Autodesk Inventor part; units mm, degrees
ref_plane "YZ Plane" through (0, 0, 0) normal (1, 0, 0) x (0, 1, 0)
ref_plane "XZ Plane" through (0, 0, 0) normal (0, 1, 0) x (-1, 0, 0)
ref_plane "XY Plane" through (0, 0, 0) normal (0, 0, 1) x (1, 0, 0)
sketch "Szkic1" plane through (0, 0, 0) normal (0, 1, 0) x (-1, 0, 0)
  line L0 (0, 0) -> (0, -97)
  line L1 (0, -97) -> (70, -97)
  line L2 (70, -97) -> (70, 0)
  line L3 (70, 0) -> (0, 0)
  line L4 (70, 0) -> (85, 0)
  line L5 (85, 0) -> (85, -97)
  line L6 (85, -97) -> (70, -97)
  line L7 (0, -97) -> (-15, -97)
  line L8 (-15, -97) -> (-15, 0)
  line L9 (-15, 0) -> (0, 0)
  line L10 (70, 0) -> (70, -25)
  line L11 (70, -25) -> (0, -25)
  line L12 (70, -97) -> (70, -72)
  line L13 (70, -72) -> (0, -72)
  line L14 (70, -48.5) -> (70, -72.5)
  line L15 (70, -48.5) -> (70, -24.5)
  line L16 (0, -48.5) -> (0, -72.5)
  line L17 (0, -48.5) -> (0, -24.5)
  dimension "d0" = 97
  dimension "d1" = 70
  dimension "d2" = 15
  dimension "d3" = 15
  dimension "d4" = 25
  dimension "d5" = 25
  dimension "d6" = 24
  dimension "d7" = 24
  dimension "d8" = 24
  dimension "d9" = 24
extrude "Wyciągnięcie proste1" add sketch "Szkic1" along normal blind 40 contours L0 L7 L8 L9 | L4 L5 L6 L2
sketch "Szkic2" plane through (0, 40, 0) normal (0, 1, 0) x (1, 0, 0)
  point P0 (0, 0)
sketch "Szkic3" plane through (0, 0, 0) normal (0, -1, 0) x (1, 0, 0)
  line L0 (-70, 0) -> (-70, -97)
  line L1 (-70, 0) -> (-70, -22)
  line L2 (-70, -22) -> (0, -22)
  line L3 (0, -97) -> (0, 0)
  line L4 (0, -22) -> (0, 0)
  line L5 (0, 0) -> (-70, 0)
  line L6 (-70, -97) -> (-70, -75)
  line L7 (-70, -75) -> (0, -75)
  line L8 (0, -97) -> (-70, -97)
  dimension "d12" = 22
  dimension "d13" = 22
extrude "Wyciągnięcie proste2" add sketch "Szkic3" against normal blind 30 contours L5 L3 L2 L0 | L7 L3 L8 L0
sketch "Szkic4" plane through (-85, 0, -97) normal (-1, 0, 0) x (0, 0, 1)
  line L0 (0, 0) -> (97, 0)
  line L1 (0, 0) -> (48.5, 0)
  line L2 (48.5, 0) -> (72.5, 0)
  line L3 (75, 0) -> (22, 0)
  line L4 (48.5, 0) -> (24.5, 0)
  line L5 (0, 0) -> (0, 40)
  line L6 (24.5, 0) -> (0, 0)
  line L7 (24.5, 0) -> (24.5, 15.2326)
  line L8 (24.5, 0) -> (39.7326, 0) construction
  line L9 (24.5, 0) -> (24.5, 20)
  circle A0 centre (24.5, 20) radius 20
  line L10 (24.5, 20) -> (72.5, 20)
  circle A1 centre (72.5, 20) radius 20
  dimension "d16" = 48.5
  dimension "d17" = 24
  dimension "d18" = 24
  dimension "d19" = 90
  dimension "d20" = 20
  dimension "d21" = 48
properties part number "podwozie"
Design review of the part built by this model. Coordinates are the model's own, in mm. A direction names the side the tool comes from. Coordinates: 2 decimals unless noted, no trailing zeros. Loops run counter-clockwise (first coordinate to the right, second up) from the corner with the lowest first, then second, coordinate; pieces in that order, holes last. Notation, with made-up numbers: (15, 32) - (74, 32) arc R17 ccw to (74, 45) - close; hole circle Ø11 at (77, 24). An arc over 180 degrees is marked (long way). Use CSV: the item, a comma, the result in double quotes. Start each with the question number.
1. Add section D-D on z = -13. Give the boundary of the cut face in (x, y).
2. Add section B-B on z = -63. Give the boundary of the cut face in (x, y), plus the area to 3 significant figures.
3. For faces 1 (the flat face through (-35, 30, -11)), 2 (the flat face through (0, 24, -48)), 3 (the flat face through (-34, 15, 0)), 4 (the flat face through (-35, 15, -75)), list the 3-axis set-ups (+Z, -Z, +X, -X, +Y, -Y) from which the entire face can be reached by the end or side of a thin tool; tool diameter is ignored.
4. Add section A-A on x = -67.5. Give the boundary of the cut face in (y, z).
5. Mouldability with a two-part tool opening along Z and no side actions: class faces 5 (the flat face through (-35, 15, -22)), 6 (the flat face through (15, 20, -49)), 7 (the flat face through (-70, 24, -49)), 8 (the flat face through (-36, 15, -97)) as released by +Z, released by -Z, zero draft, split by the parting line, or undercut.
6. Clearance check with a flat-ended pin moving along its axis: pin 1 (2 mm diameter, centred on x = -48.5, z = -86.5, fed in from +Y). State where the tip first meets the part, or that it passes through.
7. To check wall thickness, follow probe 1 along X at (y, z) = (36, -22.5); probe 2 along Z at (x, y) = (-11, 3.5); probe 3 along Y at (x, z) = (-11, -18.5). State the ranges of each line that lie inside material, in increasing order.
8. Add section C-C on y = 27. Give the boundary of the cut face in (x, z), plus the area to 3 significant figures.
Resolved:
1,outline,"(-85, 0) - (15, 0) - (15, 40) - (0, 40) - (0, 30) - (-70, 30) - (-70, 40) - (-85, 40) - close"
2,outline,"(-85, 0) - (-70, 0) - (-70, 40) - (-85, 40) - close; (0, 0) - (15, 0) - (15, 40) - (0, 40) - close"
2,area,"1,200 mm2"
3,face 1,"+Z, -Z, +Y"
3,face 2,"+Y"
3,face 3,"+Z, +X, -X, +Y, -Y"
3,face 4,"+Y, -Y"
4,outline,"(0, -97) - (30, -97) - (30, -75) - (0, -75) - close; (0, -22) - (30, -22) - (30, 0) - (0, 0) - close"
5,face 5,"undercut"
5,face 6,"zero draft"
5,face 7,"undercut"
5,face 8,"released by -Z"
6,pin 1,"y = 30"
7,probe 1,"-85 to -70, 0 to 15"
7,probe 2,"-97 to -75, -22 to 0"
7,probe 3,"0 to 30"
8,outline,"(-85, -97) - (15, -97) - (15, 0) - (-85, 0) - close; hole (-70, -75) - (0, -75) - (0, -22) - (-70, -22) - close"
8,area,"5,990 mm2"
